```python
from build123d import *

# Parameters (mm, degrees)
SKETCH1_R               = 12.5
BOSS_EXTRUDE4_DEPTH     = 40
CUT_EXTRUDE2_DEPTH      = 44.732139211
CUT_EXTRUDE2_DEPTH_BACK = 44.732139211
CUT_EXTRUDE6_DEPTH      = 44.73213936
CUT_EXTRUDE6_DEPTH_BACK = 44.73213936
CUT_EXTRUDE7_DEPTH      = 44.73213936
CUT_EXTRUDE7_DEPTH_BACK = 44.73213936


with BuildPart() as part:
    # Sketch1 → Boss-Extrude4 (new body)
    with BuildSketch(Plane(origin=(0, 0, 0), x_dir=(0, 0, -1), z_dir=(1, 0, 0))):
        Circle(SKETCH1_R)
    extrude(amount=BOSS_EXTRUDE4_DEPTH)

    # Sketch2 → Cut-Extrude2 (cut, two sides: drawn at the far end of the back side and taken through both)
    with BuildSketch(Plane.XY.offset(-CUT_EXTRUDE2_DEPTH_BACK)):
        with BuildLine():
            Line((5, 0), (5, 7.5))
            Line((5, 7.5), (30, 7.5))
            ThreePointArc((30, 7.5), (33.535533906, 6.035533906), (35, 2.5))
            Line((35, 2.5), (35, -2.5))
            ThreePointArc((35, -2.5), (33.535533906, -6.035533906), (30, -7.5))
            Line((30, -7.5), (5, -7.5))
            Line((5, -7.5), (5, 0))
        make_face()
    extrude(amount=CUT_EXTRUDE2_DEPTH + CUT_EXTRUDE2_DEPTH_BACK, mode=Mode.SUBTRACT)

    # Sketch4 → Cut-Extrude6 (cut, two sides: drawn at the far end of the back side and taken through both)
    with BuildSketch(Plane.XY.offset(-CUT_EXTRUDE6_DEPTH_BACK)):
        with BuildLine():
            Line((30, 12.5), (40, 12.5))
            Line((40, 12.5), (40, 2.5))
            ThreePointArc((40, 2.5), (37.071067812, 9.571067812), (30, 12.5))
        make_face()
    extrude(amount=CUT_EXTRUDE6_DEPTH + CUT_EXTRUDE6_DEPTH_BACK, mode=Mode.SUBTRACT)

    # Sketch5 → Cut-Extrude7 (cut, two sides: drawn at the far end of the back side and taken through both)
    with BuildSketch(Plane.XY.offset(-CUT_EXTRUDE7_DEPTH_BACK)):
        with BuildLine():
            Line((30, -12.5), (40, -12.5))
            Line((40, -12.5), (40, -2.5))
            ThreePointArc((40, -2.5), (37.071067812, -9.571067812), (30, -12.5))
        make_face()
    extrude(amount=CUT_EXTRUDE7_DEPTH + CUT_EXTRUDE7_DEPTH_BACK, mode=Mode.SUBTRACT)


solid = part.part
```
Geometry check sheet. Reference: the model listing, model coordinates, mm. A direction names the side the tool comes from. Coordinates: 2 decimals unless noted, no trailing zeros. Order: outer loops, then holes, each group sorted by start corner. A loop starts at its lowest first (then second) coordinate and runs counter-clockwise, first axis right, second up. Notation, with made-up numbers: M 69.25,-34.75 L 107.25,-34.75 A29 ccw 107.25,-5.75 Z; hole C 76.25,-37 d4. An arc over 180 degrees is marked long. One line per question, with ' | ' between items. Start each with the question number.
Item 1: Cross-section at A-A on y = 0. Enter the section's corners in (x, z), then the cut area to 3 significant figures.
Item 2: Draft check along X on faces 1 (the flat face through (40, 0, 0)), 2 (the flat face through (0, 0, 0)), 3 (the flat face through (5, 0, 0)). Enter one of: pulls with the +X half, pulls with the -X half, needs draft (parallel to the pull), parting line crosses it, or undercut.
Item 3: Set-up check for faces 4 (the flat face through (17, 7.5, 0)), 5 (the cylindrical face through (19.72, 8.45, 9.21)): record each of +Z, -Z, +X, -X, +Y, -Y from which the full face is reachable in a straight line by a thin tool's end or side.
Item 4: Cross-section at B-B on z = 0. Enter the section's corners in (x, y).
Item 5: Cross-section at D-D on z = 10.5. Enter the section's corners in (x, y), then the cut area to 3 significant figures.
Item 6: Gauge pin test, flat ends, axial feed: pin 1 (12 mm diameter, centred on x = 25.5, y = 4.5, fed in from -Z); pin 2 (1.5 mm diameter, centred on x = 29.5, z = -6.5, fed in from +Y); pin 3 (2 mm diameter, centred on x = 16.5, z = 2.5, fed in from -Y). Record the tip position at first contact, or that the pin passes through.
Item 7: Cross-section at C-C on x = 12. Enter the section's corners in (y, z), then the cut area to 3 significant figures.
Item 8: Material ranges on L1, parallel to X at y = 1, z = -9; L2, parallel to Y at x = 31, z = 7.75; L3, parallel to Y at x = 13, z = 0.75, recorded low to high. Write a range as [from, to].
Findings:
1) outline: M 0,-12.5 L 5,-12.5 L 5,12.5 L 0,12.5 Z; M 35,-12.5 L 40,-12.5 L 40,12.5 L 35,12.5 Z | area: 250 mm²
2) face 1: pulls with the +X half | face 2: pulls with the -X half | face 3: undercut
3) face 4: +Z, -Z | face 5: +X, -X
4) outline: M 0,-12.5 L 30,-12.5 A10 ccw 40,-2.5 L 40,2.5 A10 ccw 30,12.5 L 0,12.5 Z; hole M 5,-7.5 L 30,-7.5 A5 ccw 35,-2.5 L 35,2.5 A5 ccw 30,7.5 L 5,7.5 Z
5) outline: M 0,-6.78 L 5,-6.78 L 5,6.78 L 0,6.78 Z; M 32.58,-6.78 L 39.04,-6.78 A10 ccw 40,-2.5 L 40,2.5 A10 ccw 39.04,6.78 L 32.58,6.78 A5 cw 35,2.5 L 35,-2.5 A5 cw Z | area: 139 mm²
6) pin 1: stops at z = -10.04 | pin 2: stops at y = 11.1 | pin 3: stops at y = -12.41
7) outline: M -7.5,-10 L -7.5,10 A12.5 ccw Z; M 7.5,-10 A12.5 ccw 7.5,10 Z | area: 140 mm²
8) L1: x = [0, 5], [35, 40] | L2: y = [-9.81, -7.4], [7.4, 9.81] | L3: y = [-12.48, -7.5], [7.5, 12.48]
